Model file for the job. Use its own axes, mm. Face numbers are marked on the shaded views. A direction names the side the tool comes from. Coordinates: 2 decimals unless noted, no trailing zeros. Write each loop counter-clockwise with the first axis right and the second up, starting at its lowest first coordinate (ties: lowest second). Pieces come first, ordered by that corner, then holes. Notation, with made-up numbers: M 5,28.25 L 58,28.25 A6 ccw 58,34.25 Z; hole C -27.75,13 d5. An arc over 180 degrees is marked long. Put each result on its own line as item: value. Start each with the question number.
Q1. Drop flat-ended pins along their axis: pin 1 (2 mm diameter, centred on x = 2.5, z = 12.5, fed in from -Y); pin 2 (3 mm diameter, centred on x = 34, y = -14, fed in from -Z); pin 3 (12 mm diameter, centred on x = 30.5, y = -24.5, fed in from +Z); pin 4 (4 mm diameter, centred on y = -21, z = -3.5, fed in from +X). Give the stop position or say it passes through.
Q2. Pull direction X, two halves, no side cores. Call the marked faces 4, 5 and 6: pulls with the +X half, pulls with the -X half, needs draft (parallel to the pull), parting line crosses it, or undercut.
Q3. Which spindle directions (+Z, -Z, +X, -X, +Y, -Y) get a long thin tool onto all of the face, cutting with end or side? Do the marked faces 1, 2 and 3. Say none if no direction does.
Q4. Cut at B-B (z = -1.5). Write the cut outline in (x, y).
Q5. Cut at A-A (x = 34.5). Write the cut outline in (y, z), then the cut area to 3 significant figures.
Q6. Drill centre lines: line 1 along X through (y, z) = (-7, -3.5); line 2 along X through (y, z) = (-3.75, 12.5); line 3 along X through (y, z) = (-28.5, -18.5). Where is each one in solid material? Low to high.
Q7. Cut at C-C (y = -1.75). Write the cut outline in (x, z).
```python
from build123d import *

# Parameters (mm, degrees)
F0_R     = 2.963143
F0_R_2   = 3.00478
F0_R_3   = 5.870107
F0_R_4   = 10.138773
F0_R_5   = 2.878059
F0_R_6   = 2.878057
F1_DEPTH = 30


with BuildPart() as f1:
    # F0 (on Front) → F1 (new body)
    with BuildSketch(Plane.XZ):
        Polygon((0, 17.412249), (-40.724516, 17.124442), (-40.724516, -26.622033), (-4.431914, -26.622033), (-1.612007, -26.622033), (47.344048, -26.622033), (47.344048, -7.339047), (0, -7.339047), (0, 11.686382), (0, 15.079555), align=None)
        with Locations((-36.695234, -21.729333)):
            Circle(F0_R, mode=Mode.SUBTRACT)
        with Locations((-6.187823, -23.456169)):
            Circle(F0_R_2, mode=Mode.SUBTRACT)
        with Locations((33.81718, -17.124442)):
            Circle(F0_R_3, mode=Mode.SUBTRACT)
        with Locations((-19.714694, -3.885378)):
            Circle(F0_R_4, mode=Mode.SUBTRACT)
        with Locations((-36.983039, 13.095162)):
            Circle(F0_R_5, mode=Mode.SUBTRACT)
        with Locations((-5.612212, 13.382968)):
            Circle(F0_R_6, mode=Mode.SUBTRACT)
        with BuildLine():
            Line((-1.612007, -26.622033), (-4.431914, -26.622033))
            ThreePointArc((-4.431914, -26.622033), (-3.021961, -26.921809), (-1.612007, -26.622033))
        make_face()
        with BuildLine():
            ThreePointArc((0, 11.686382), (0.48361, 13.382968), (0, 15.079555))
            Line((0, 15.079555), (0, 11.686382))
        make_face()
    extrude(amount=F1_DEPTH)


solid = f1.part
```
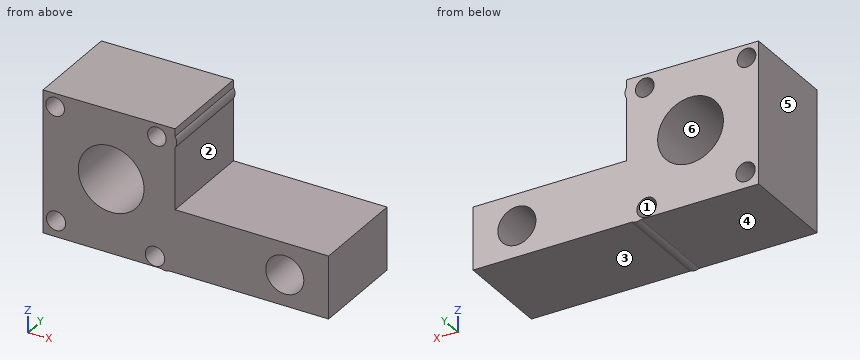
Computed values:
1. pin 1: through
1. pin 2: z = -26.62
1. pin 3: z = -7.34
1. pin 4: x = 0
2. face 4: needs draft
2. face 5: pulls with the -X half
2. face 6: undercut
3. face 1: +Y, -Y
3. face 2: +X, +Y, -Y
3. face 3: -Z, +X, +Y, -Y
4. outline: M -40.72,-30 L -29.57,-30 L -29.57,0 L -40.72,0 Z; M -9.86,-30 L 0,-30 L 0,0 L -9.86,0 Z
5. outline: M -30,-26.62 L 0,-26.62 L 0,-22.95 L -30,-22.95 Z; M -30,-11.29 L 0,-11.29 L 0,-7.34 L -30,-7.34 Z
5. area: 229 mm2
6. line 1: -40.72 to -29.85, -9.58 to 0
6. line 2: -40.72 to -39.8, -34.17 to -8.35, -2.87 to 0.36
6. line 3: -40.72 to 28.11, 39.52 to 47.34
7. outline: M -40.72,-26.62 L -4.43,-26.62 A3.47 ccw -1.61,-26.62 L 47.34,-26.62 L 47.34,-7.34 L 0,-7.34 L 0,11.69 A3.22 ccw 0,15.08 L 0,17.41 L -40.72,17.12 Z; hole C -36.98,13.1 d5.76; hole C -36.7,-21.73 d5.93; hole C -19.71,-3.89 d20.28; hole C -6.19,-23.46 d6.01; hole C -5.61,13.38 d5.76; hole C 33.82,-17.12 d11.74
